Autodesk Inventor part; units mm, degrees
ref_plane "YZ Plane" through (0, 0, 0) normal (1, 0, 0) x (0, 1, 0)
ref_plane "XZ Plane" through (0, 0, 0) normal (0, 1, 0) x (-1, 0, 0)
ref_plane "XY Plane" through (0, 0, 0) normal (0, 0, 1) x (1, 0, 0)
sketch "Sketch1" plane through (0, 0, 0) normal (1, 0, 0) x (0, 1, 0)
  line L0 (2812.3869, 0) -> (2812.3869, -5171.1623) construction
  line L1 (2812.3869, -5171.1623) -> (0, -5171.1623) construction
  line L2 (0, -5171.1623) -> (0, 0) construction
  line L3 (0, 0) -> (2812.3869, 0) construction
  point P0 (0, 0)
sketch "Sketch2" plane through (0, 0, 0) normal (1, 0, 0) x (0, 1, 0)
  arc A0 (753.391, -1473.8258) -> (725.6652, -1208.6158) centre (409.0296, -1375.7721) ccw
  arc A1 (692.5478, -1452.6934) -> (667.2559, -1239.5627) centre (430.475, -1375.7271) ccw
  arc A2 (725.6652, -1208.6158) -> (667.2559, -1239.5627) centre (696.4374, -1224.0456) ccw
  arc A3 (692.5478, -1452.6934) -> (753.391, -1473.8258) centre (722.3676, -1464.9922) ccw
  circle A4 centre (696.4374, -1222.1798) radius 15
  circle A5 centre (727.5117, -1457.7884) radius 15
  point P0 (0, 0)
  dimension "d4" = 30
  dimension "d5" = 30
extrude "Extrusion1" add sketch "Sketch2" along normal mid plane 30
fillet "Fillet1" radius 2 8 edges at (15, 765.1382, -1338.5435) (15, 680.964, -1194.8409) (15, 701.7128, -1343.5398) (15, 711.7843, -1495.4631) (-15, 765.1382, -1338.5435) (-15, 711.7843, -1495.4631) (-15, 701.7128, -1343.5398) (-15, 680.964, -1194.8409)
properties part number "Lankarm_kort"
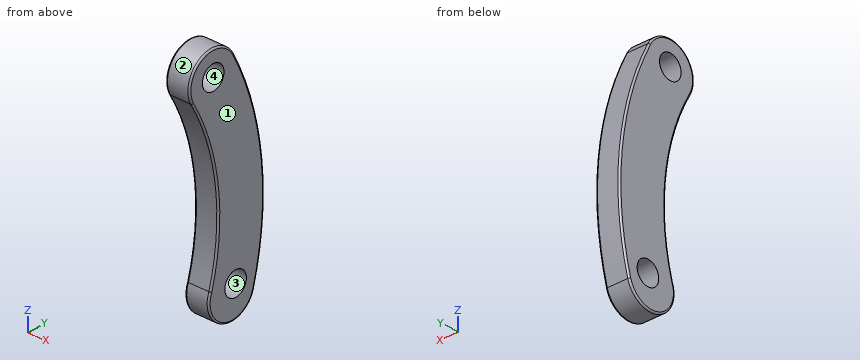
Verification items for the finished model (mm, model axes). Face numbers are marked on the shaded views. Coordinates: 2 decimals unless noted, no trailing zeros. Order: outer loops, then holes, each group sorted by start corner. A loop starts at its lowest first (then second) coordinate and runs counter-clockwise, first axis right, second up.
1. Go/stop test with flat-tipped pins: pin 1 Ø5 at (x, y) = (9, 736) entering from -Z; pin 2 Ø4 at (x, y) = (6, 683.5) entering from +Z; pin 3 Ø5 at (x, z) = (-11.5, -1296) entering from -Y; pin 4 Ø12 at (y, z) = (699.5, -1390) entering from +X. Record where each tip stops, or that it passes through.
Results found:
pin 1: stops at z = -1495.27
pin 2: stops at z = -1192.86
pin 3: stops at y = 690.95
pin 4: stops at x = 15
2. Release check for a two-part mould opening along Z. For the marked faces 1, 2, 3 and 4 record: +Z half, -Z half, draft (parallel to the pull), parting line (faces both ways), or undercut.
Results found:
face 1: draft
face 2: parting line
face 3: undercut
face 4: undercut
3. Scan lines: line 1 (Z direction, x = -3, y = 719); line 2 (Z direction, x = -1.5, y = 704.5); line 3 (Y direction, x = 2, z = -1356.5). Record each from-to range of solid material in increasing order.
Results found:
line 1: z = -1497.07 to -1470.14, -1445.44 to -1199.89
line 2: z = -1491.85 to -1234.83, -1209.53 to -1191.99
line 3: y = 702.94 to 766.56
4. Sectioned sample at A-A, the plane x = 4. Record the cut outline in (y, z), and give its area (3 significant figures).
Results found:
outline: (667.26, -1239.56) arc R273.14 cw to (692.55, -1452.69) arc R32.26 ccw (long way) to (753.39, -1473.83) arc R358.05 ccw to (725.67, -1208.62) arc R33.05 ccw to start; hole circle Ø30 at (696.44, -1222.18); hole circle Ø30 at (727.51, -1457.79)
area: 17,900 mm2
5. Sectioned sample at B-B, the plane y = 701. Give the number of separate pieces and of enclosed holes in the cut face, and give its area (3 significant figures).
Results found:
separate pieces: 3
enclosed holes: 0
area: 5,790 mm2
